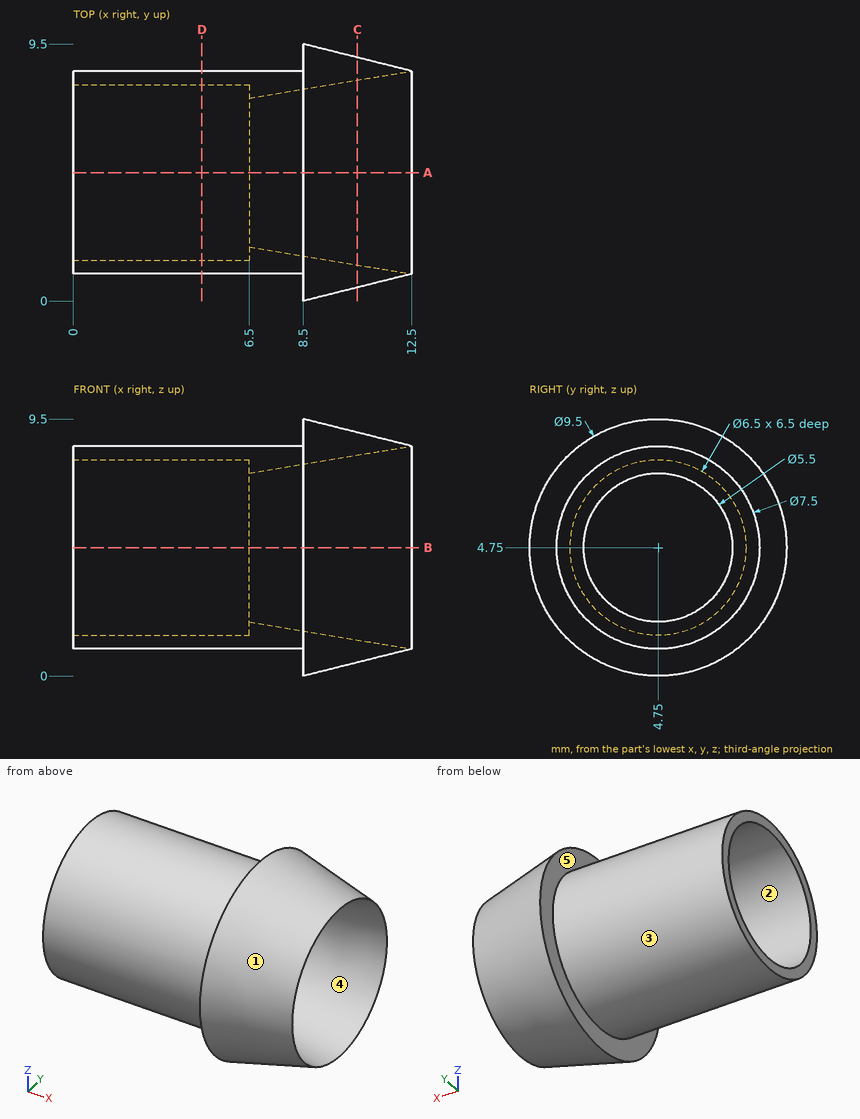
For this review, use the dimensioned drawing (mm, ordinates from the lowest corner) and the shaded views. A direction names the side the tool comes from. Give positions to 0.01 mm unless a question says otherwise; leave off trailing zeros. Write each loop counter-clockwise with the first axis right and the second up, starting at its lowest first coordinate (ties: lowest second). Pieces come first, ordered by that corner, then holes. Notation, with made-up numbers: M 51,20.5 L 92,20.5 A20 cw 92,36.5 Z; hole C 15,46.5 d11. An arc over 180 degrees is marked long. Answer as a JSON object with one key per item and string values. Group by question number.
Item 1: For pin 1 Ø5 at (y, z) = (2.5, 4) entering from -X; pin 2 Ø5 at (x, y) = (2, 6) entering from +Z; pin 3 Ø4 at (x, z) = (5.5, 3.5) entering from -Y; pin 4 Ø5 at (x, z) = (11, 8) entering from -Y, all flat-tipped, find the tip position at first contact; note any pin that passes through.
Item 2: Consider section D-D on x = 4.75. Write out the cut boundary in (y, z), plus the area to 3 significant figures.
Item 3: Consider section A-A on y = 4.75. Write out the cut boundary in (x, z), plus the area to 3 significant figures.
Item 4: For probe 1 along Y at (x, z) = (3.5, 4.75); probe 2 along Y at (x, z) = (11.25, 4.5), list the stretches that pass through material, from the lowest coordinate up. Write a range as [from, to].
Item 5: Draft analysis for pull direction Z (two halves, no side actions). For the marked faces 3, 4 and 5, state which applies: +Z half, -Z half, draft (parallel to the pull), parting line (faces both ways), or undercut.
Item 6: Tool access review of the marked faces 1 and 2: name each direction out of +Z, -Z, +X, -X, +Y, -Y from which nothing blocks a thin tool from reaching the whole face with its end or side.
Item 7: Consider section C-C on x = 10.5. Write out the cut boundary in (y, z).
Check result:
{
 "1": {"pin 1": "stops at x = 0", "pin 2": "stops at z = 8.5", "pin 3": "stops at y = 1", "pin 4": "stops at y = 0.42"},
 "2": {"outline": "C 4.75,4.75 d7.5; hole C 4.75,4.75 d6.5", "area": "11.0 mm^2"},
 "3": {"outline": "M 0,1 L 8.5,1 L 8.5,0 L 12.5,1 L 6.5,2 L 6.5,1.5 L 0,1.5 Z; M 0,8 L 6.5,8 L 6.5,7.5 L 12.5,8.5 L 8.5,9.5 L 8.5,8.5 L 0,8.5 Z", "area": "16.5 mm^2"},
 "4": {"probe 1": "y = [1, 1.5], [8, 8.5]", "probe 2": "y = [0.7, 1.22], [8.28, 8.8]"},
 "5": {"face 3": "parting line", "face 4": "undercut", "face 5": "draft"},
 "6": {"face 1": "+X", "face 2": "-X"},
 "7": {"outline": "C 4.75,4.75 d8.5; hole C 4.75,4.75 d6.83"}
}
